```python
from build123d import *

# Parameters (mm, degrees)
CYLINDER005_R               = 1.25
CYLINDER005_DEPTH           = 10
BOX007_W                    = 23
BOX007_H                    = 2.75
BOX007_DEPTH                = 2
CYLINDER002_W               = 4
CYLINDER002_H               = 26
CYLINDER002_ANGLE           = 195
CYLINDER002_PLACEMENT_ANGLE = 105


with BuildPart() as b_so:
    # Cylinder005 → Cylinder005 (new body)
    with BuildSketch(Plane(origin=(41, 5, 4), x_dir=(1, 0, 0), z_dir=(0, 0, 1))):
        Circle(CYLINDER005_R)
    extrude(amount=CYLINDER005_DEPTH)


with BuildPart() as o001:
    # Box007 → Box007 (new body)
    with BuildSketch(Plane(origin=(40, 5, 10), x_dir=(0, 1, 0), z_dir=(0, 0, 1))):
        with Locations((11.5, 1.375)):
            Rectangle(BOX007_W, BOX007_H)
    extrude(amount=BOX007_DEPTH)


with BuildPart() as cut002_o:
    # Cylinder002 → Cylinder002 (revolve)
    with BuildSketch(Plane.XZ):
        with Locations((2, 13)):
            Rectangle(CYLINDER002_W, CYLINDER002_H)
    revolve(axis=Axis((0, 0, 0), (0, 0, 1)), revolution_arc=CYLINDER002_ANGLE)


with BuildPart() as cut002_o_1:
    # Cylinder002 placement: moved
    add(cut002_o.part.moved(Location((40, 5, -14))).rotate(Axis((40, 5, -14), (0, 0, -1)), CYLINDER002_PLACEMENT_ANGLE))

    # Fusion004: union O001
    add(o001.part)

    # Cut002: cut B_SO
    add(b_so.part, mode=Mode.SUBTRACT)


with BuildPart() as cut002_o_2:
    # Cut002 placement: moved
    add(cut002_o_1.part.moved(Location((40, 5, 0))))


solid = cut002_o_2.part
```
Part model, mm, in its own coordinate system. A direction names the side the tool comes from. Round coordinates to 2 decimals unless told otherwise and drop trailing zeros. Loops run counter-clockwise (first coordinate to the right, second up) from the corner with the lowest first, then second, coordinate; pieces in that order, holes last.
1. 3-axis set-ups, long thin cutter, end or side, ignore diameter. For faces 1 (the face through (77.25, 21, 11)), 2 (the face through (79, 21, 10)), 3 (the face through (79, 19, 12)), 4 (the face through (81, 10, 4)), 5 (the face through (80, 23, 11)): which of +Z, -Z, +X, -X, +Y, -Y reach the whole face in a straight line?
Solutions:
face 1: +Z, -Z, -X, +Y, -Y
face 2: -Z, -X, +Y
face 3: +Z, +X, -X, +Y, -Y
face 4: +Z
face 5: +Z, -Z, +X, +Y
2. Slice it at A-A (x = 81). Give the cut face in (y, z).
Solutions:
outline: (6.13, -14) - (13.87, -14) - (13.87, 12) - (11.25, 12) - (11.25, 4) - (8.75, 4) - (8.75, 12) - (6.13, 12) - close
3. Slice it at D-D (z = 8.5). Give the cut face in (x, y).
Solutions:
outline: (78.96, 6.14) arc R4 ccw (long way) to (80, 14) - (80, 10.75) arc R1.25 cw (long way) to (79.86, 9.48) - close
4. Slice it at B-B (y = 20). Give the cut face in (x, z).
Solutions:
outline: (77.25, 10) - (80, 10) - (80, 12) - (77.25, 12) - close
5. Slice it at C-C (z = -11.75). Give the cut face in (x, y), and give its area (3 significant figures).
Solutions:
outline: (78.96, 6.14) arc R4 ccw (long way) to (80, 14) - (80, 10) - close
area: 27.2 mm2
6. Drill centre lines: line 1 along X through (y, z) = (10, 5.75); line 2 along Z through (x, y) = (81.5, 10.25); line 3 along Y through (x, z) = (80.5, 6.75). Where is each one in solid material? Low to high.
Solutions:
line 1: x = 82.25 to 84
line 2: z = -14 to 4
line 3: y = 6.03 to 8.85, 11.15 to 13.97
7. Two-plate mould, pull along Y, no slides. Class faces 6 (the face through (79, 33, 11)), 7 (the face through (80, 12, -2)), 8 (the face through (79, 10, 11)): pulls with the +Y half, pulls with the -Y half, needs draft (parallel to the pull), parting line crosses it, or undercut.
Solutions:
face 6: pulls with the +Y half
face 7: needs draft
face 8: undercut
8. Flat gauge pins, fed straight in: pin 1 (1.5 mm diameter, centred on x = 81, y = 10, fed in from +Z); pin 2 (0.6 mm diameter, centred on y = 24.5, z = 11.5, fed in from +X); pin 3 (1.6 mm diameter, centred on x = 78.5, z = 11, fed in from -Y); pin 4 (1 mm diameter, centred on x = 78, z = 8, fed in from -Y). Where does each tip first touch, or does it go through?
Solutions:
pin 1: stops at z = 4
pin 2: stops at x = 80
pin 3: stops at y = 6.06
pin 4: passes through
